Drawing for the job (mm, zero at the part's lowest x, y, z). A direction names the side the tool comes from. Round coordinates to 2 decimals unless told otherwise and drop trailing zeros. Write each loop counter-clockwise with the first axis right and the second up, starting at its lowest first coordinate (ties: lowest second). Pieces come first, ordered by that corner, then holes.
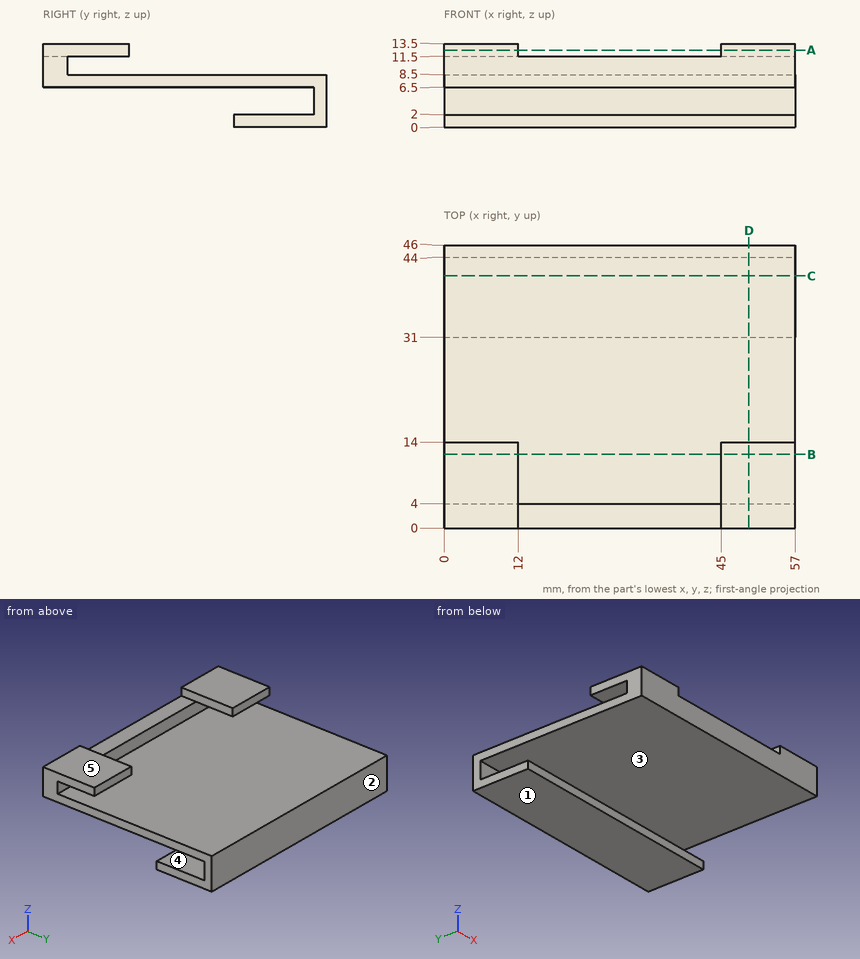
1) Cut at A-A on z = 12.5. List the corners of the cut face in (x, y).
2) Cut at D-D on x = 49.5. List the corners of the cut face in (y, z), and give its area (3 significant figures).
3) Cut at C-C on y = 41. List the corners of the cut face in (x, z), and give its area (3 significant figures).
4) Wall check: probe 1 along Z at (x, y) = (50, 32); probe 2 along Y at (x, z) = (47, 10.75); probe 3 along Z at (x, y) = (22, 29). Give the ranges that are in metal, low to high.
5) Pull direction Z, two halves, no side cores. Call the marked faces 1, 2 and 3: released by +Z, released by -Z, zero draft, split by the parting line, or undercut.
6) Flat gauge pins, fed straight in: pin 1 Ø1.5 at (x, z) = (20.5, 5.5) entering from -Y; pin 2 Ø22 at (x, y) = (34.5, 19.5) entering from -Z; pin 3 Ø6.5 at (x, y) = (37, 37.5) entering from +Z. Where does each tip first touch, or does it go through?
7) Cut at B-B on y = 12. List the corners of the cut face in (x, z), and give its area (3 significant figures).
8) Which spindle directions (+Z, -Z, +X, -X, +Y, -Y) get a long thin tool onto all of the face, cutting with end or side? Do the marked faces 4 and 5. Say none if no direction does.
Result sheet:
1. outline: (0, 0) - (12, 0) - (12, 14) - (0, 14) - close; (45, 0) - (57, 0) - (57, 14) - (45, 14) - close
2. outline: (0, 6.5) - (44, 6.5) - (44, 2) - (31, 2) - (31, 0) - (46, 0) - (46, 8.5) - (4, 8.5) - (4, 11.5) - (14, 11.5) - (14, 13.5) - (0, 13.5) - close
2. area: 171 mm2
3. outline: (0, 0) - (57, 0) - (57, 2) - (0, 2) - close; (0, 6.5) - (57, 6.5) - (57, 8.5) - (0, 8.5) - close
3. area: 228 mm2
4. probe 1: z = 0 to 2, 6.5 to 8.5
4. probe 2: y = 0 to 4
4. probe 3: z = 6.5 to 8.5
5. face 1: released by -Z
5. face 2: zero draft
5. face 3: undercut
6. pin 1: stops at y = 44
6. pin 2: stops at z = 6.5
6. pin 3: stops at z = 8.5
7. outline: (0, 6.5) - (57, 6.5) - (57, 8.5) - (0, 8.5) - close; (0, 11.5) - (12, 11.5) - (12, 13.5) - (0, 13.5) - close; (45, 11.5) - (57, 11.5) - (57, 13.5) - (45, 13.5) - close
7. area: 162 mm2
8. face 4: +X, -X, -Y
8. face 5: +Z, +X, -X, +Y, -Y
